from build123d import *

# Parameters (mm, degrees)
EXTRUDE_1_DEPTH = 2
EXTRUDE_2_DEPTH = 2
OTHER_START     = 1
OTHER_1_DEPTH   = 1


# Read off the part's stored shape, not the designer's step: Полость1
with BuildPart() as part:
    # Эскиз1 → Бобышка-Вытянуть1 (new body)
    with BuildSketch(Plane.XY):
        with BuildLine():
            Line((-4.017219652, 1.762254744), (-38.034439304, 16.684766311))
            ThreePointArc((-38.034439304, 16.684766311), (-46.743488079, 24.061279464), (-50, 35))
            Line((-50, 35), (-50, 150))
            Line((-50, 150), (50, 150))
            Line((50, 150), (50, 35))
            ThreePointArc((50, 35), (46.743488079, 24.061279464), (38.034439304, 16.684766311))
            Line((38.034439304, 16.684766311), (4.017219652, 1.762254744))
            ThreePointArc((4.017219652, 1.762254744), (0, 0.919871589), (-4.017219652, 1.762254744))
        make_face()
    extrude(amount=EXTRUDE_1_DEPTH)

    # Эскиз2 → Бобышка-Вытянуть2 (add)
    with BuildSketch(Plane.XY.offset(2)):
        with BuildLine():
            Line((50, 150), (-50, 150))
            Line((-50, 150), (-50, 35))
            ThreePointArc((-50, 35), (-46.743488079, 24.061279464), (-38.034439304, 16.684766311))
            Line((-38.034439304, 16.684766311), (-4.017219652, 1.762254744))
            ThreePointArc((-4.017219652, 1.762254744), (0, 0.919871589), (4.017219652, 1.762254744))
            Line((4.017219652, 1.762254744), (38.034439304, 16.684766311))
            ThreePointArc((38.034439304, 16.684766311), (46.743488079, 24.061279464), (50, 35))
            Line((50, 35), (50, 150))
        make_face()
        with BuildLine():
            Line((46, 146), (-46, 146))
            Line((-46, 146), (-46, 35))
            ThreePointArc((-46, 35), (-43.394790463, 26.249023571), (-36.427551443, 20.347813049))
            Line((-36.427551443, 20.347813049), (-2.410331791, 5.425301482))
            ThreePointArc((-2.410331791, 5.425301482), (0, 4.919871589), (2.410331791, 5.425301482))
            Line((2.410331791, 5.425301482), (36.427551443, 20.347813049))
            ThreePointArc((36.427551443, 20.347813049), (43.394790463, 26.249023571), (46, 35))
            Line((46, 35), (46, 146))
        make_face(mode=Mode.SUBTRACT)
    extrude(amount=EXTRUDE_2_DEPTH)

    # Полость1 outline → Полость1 (cut)
    with BuildSketch(Plane.XY.offset(OTHER_START)):
        with BuildLine():
            ThreePointArc((11.745635367, 75.156774095), (20.994280281, 69.854105541), (11.31836185, 65.378356547))
            ThreePointArc((11.31836185, 65.378356547), (5.115095453, 80.478737769), (3, 96.666029027))
            Line((3, 96.666029027), (4.5, 126.216029027))
            ThreePointArc((4.5, 126.216029027), (3.337458241, 132.579990058), (0, 138.121909927))
            ThreePointArc((0, 138.121909927), (-3.33745824, 132.579990058), (-4.5, 126.216029027))
            Line((-4.5, 126.216029027), (-3, 96.666029027))
            ThreePointArc((-3, 96.666029027), (-5.115095453, 80.478737769), (-11.31836185, 65.378356547))
            ThreePointArc((-11.31836185, 65.378356547), (-20.994280281, 69.854105541), (-11.745635367, 75.156774095))
            Line((-11.745635367, 75.156774095), (-13.469683479, 99.811810763))
            ThreePointArc((-13.469683479, 99.811810763), (-20.328911117, 119.444533663), (-36, 133.116029027))
            Line((-36, 133.116029027), (-36, 43.116029027))
            Line((-36, 43.116029027), (-16.549961479, 43.116029027))
            ThreePointArc((-16.549961479, 43.116029027), (-12.036010614, 31.549603352), (-3.567460781, 22.469866625))
            ThreePointArc((-3.567460781, 22.469866625), (-1.525407448, 20.507840011), (0, 18.121909927))
            ThreePointArc((0, 18.121909927), (1.525407448, 20.507840011), (3.567460781, 22.469866625))
            ThreePointArc((3.567460781, 22.469866625), (12.036010614, 31.549603352), (16.549961479, 43.116029027))
            Line((16.549961479, 43.116029027), (36, 43.116029027))
            Line((36, 43.116029027), (36, 133.116029027))
            ThreePointArc((36, 133.116029027), (20.328911117, 119.444533663), (13.469683479, 99.811810763))
            Line((13.469683479, 99.811810763), (11.745635367, 75.156774095))
        make_face()
        with BuildLine():
            ThreePointArc((-3, 29.83417227), (-7.667449376, 35.941229982), (-10.424893162, 43.116029027))
            Line((-10.424893162, 43.116029027), (-3, 43.116029027))
            Line((-3, 43.116029027), (-3, 29.83417227))
        make_face(mode=Mode.SUBTRACT)
        with BuildLine():
            ThreePointArc((-15.840643779, 58.145510324), (-16.78364457, 53.674469292), (-17.1, 49.116029027))
            Line((-17.1, 49.116029027), (-30, 49.116029027))
            Line((-30, 49.116029027), (-30, 67.116029027))
            Line((-30, 67.116029027), (-26.618950039, 67.116029027))
            ThreePointArc((-26.618950039, 67.116029027), (-22.676452369, 60.892576365), (-15.840643779, 58.145510324))
        make_face(mode=Mode.SUBTRACT)
        with BuildLine():
            ThreePointArc((-9.793333333, 57.413777048), (-4.715017619, 54.57423386), (-2.7, 49.116029027))
            Line((-2.7, 49.116029027), (-11.1, 49.116029027))
            ThreePointArc((-11.1, 49.116029027), (-10.771332925, 53.316029027), (-9.793333333, 57.413777048))
        make_face(mode=Mode.SUBTRACT)
        with BuildLine():
            Line((3, 29.83417227), (3, 43.116029027))
            Line((3, 43.116029027), (10.424893162, 43.116029027))
            ThreePointArc((10.424893162, 43.116029027), (7.667449376, 35.941229982), (3, 29.83417227))
        make_face(mode=Mode.SUBTRACT)
        with BuildLine():
            ThreePointArc((2.7, 49.116029027), (4.715017619, 54.57423386), (9.793333333, 57.413777048))
            ThreePointArc((9.793333333, 57.413777048), (10.771332925, 53.316029027), (11.1, 49.116029027))
            Line((11.1, 49.116029027), (2.7, 49.116029027))
        make_face(mode=Mode.SUBTRACT)
        with BuildLine():
            ThreePointArc((0, 79.005460407), (2.806605948, 70.695071551), (6.654810678, 62.812754617))
            ThreePointArc((6.654810678, 62.812754617), (3.005032266, 61.025332003), (0, 58.289359938))
            ThreePointArc((0, 58.289359938), (-3.005032266, 61.025332003), (-6.654810678, 62.812754617))
            ThreePointArc((-6.654810678, 62.812754617), (-2.806605948, 70.695071551), (0, 79.005460407))
        make_face(mode=Mode.SUBTRACT)
        with BuildLine():
            ThreePointArc((17.1, 49.116029027), (16.78364457, 53.674469292), (15.840643779, 58.145510324))
            ThreePointArc((15.840643779, 58.145510324), (22.676452369, 60.892576365), (26.618950039, 67.116029027))
            Line((26.618950039, 67.116029027), (30, 67.116029027))
            Line((30, 67.116029027), (30, 49.116029027))
            Line((30, 49.116029027), (17.1, 49.116029027))
        make_face(mode=Mode.SUBTRACT)
        with BuildLine():
            ThreePointArc((-18.216224905, 81.676993406), (-23.564060467, 78.521793021), (-26.618950039, 73.116029027))
            Line((-26.618950039, 73.116029027), (-30, 73.116029027))
            Line((-30, 73.116029027), (-30, 121.661547275))
            ThreePointArc((-30, 121.661547275), (-22.554855421, 111.225521288), (-19.413361995, 98.796851397))
            Line((-19.413361995, 98.796851397), (-18.216224905, 81.676993406))
        make_face(mode=Mode.SUBTRACT)
        with BuildLine():
            ThreePointArc((19.413361995, 98.796851397), (22.554855421, 111.225521288), (30, 121.661547275))
            Line((30, 121.661547275), (30, 73.116029027))
            Line((30, 73.116029027), (26.618950039, 73.116029027))
            ThreePointArc((26.618950039, 73.116029027), (23.564060467, 78.521793021), (18.216224905, 81.676993406))
            Line((18.216224905, 81.676993406), (19.413361995, 98.796851397))
        make_face(mode=Mode.SUBTRACT)
    extrude(amount=OTHER_1_DEPTH, mode=Mode.SUBTRACT)


solid = part.part
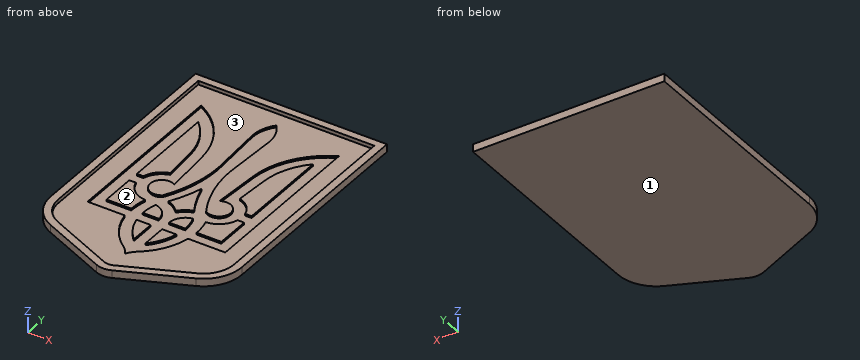
The model under review builds one solid part; all positions refer to its coordinate system, in mm. Face numbers are marked on the shaded views. Coordinates: 2 decimals unless noted, no trailing zeros. Order: outer loops, then holes, each group sorted by start corner. A loop starts at its lowest first (then second) coordinate and runs counter-clockwise, first axis right, second up. Notation, with made-up numbers: (87, 37.5) -> (117, 37.5) arc R32 ccw to (117, 71.5) -> close; hole circle Ø2 at (86, -40). An arc over 180 degrees is marked (long way). Answer in a Markdown table with one row per item.
(1) Consider section B-B (x = -33). Write out the cut boundary in (y, z).
Answers:
| item | result |
|---|---|
| outline | (14.48, 0) -> (150, 0) -> (150, 4) -> (146, 4) -> (146, 2) -> (131.47, 2) -> (131.47, 1) -> (43.12, 1) -> (43.12, 2) -> (18.84, 2) -> (18.84, 4) -> (14.48, 4) -> close |
(2) The part is to be moulded in two halves that separate along Y. For the marked faces 1, 2 and 3, say which applies: +Y half, -Y half, draft (parallel to the pull), parting line (faces both ways), or undercut.
Answers:
| item | result |
|---|---|
| face 1 | draft |
| face 2 | undercut |
| face 3 | undercut |
(3) Wall thickness on line 1 along X through (y, z) = (80.5, 2.35); line 2 along X through (y, z) = (59.5, 1.8); line 3 along X through (y, z) = (37, 1.85): over which ranges is each line inside the solid? List them lowest first.
Answers:
| item | result |
|---|---|
| line 1 | -50 to -46, 46 to 50 |
| line 2 | -50 to -36, -30 to -20.59, -1.12 to 1.12, 20.59 to 30, 36 to 50 |
| line 3 | -50 to -14.8, -8.23 to -3, 3 to 8.23, 14.8 to 50 |
(4) Consider section A-A (y = 41.5). Write out the cut boundary in (x, z), plus the area to 3 significant figures.
Answers:
| item | result |
|---|---|
| outline | (-50, 0) -> (50, 0) -> (50, 4) -> (46, 4) -> (46, 2) -> (16.21, 2) -> (16.21, 1) -> (10, 1) -> (10, 2) -> (3, 2) -> (3, 1) -> (-3, 1) -> (-3, 2) -> (-10, 2) -> (-10, 1) -> (-16.21, 1) -> (-16.21, 2) -> (-46, 2) -> (-46, 4) -> (-50, 4) -> close |
| area | 198 mm² |
(5) Insertion check: pin 1 (1.1 mm diameter, centred on x = 20.5, z = 1.5, fed in from -Y); pin 2 (11.5 mm diameter, centred on x = -22.5, y = 56.5, fed in from +Z); pin 3 (0.8 mm diameter, centred on x = -25, z = 1.5, fed in from -Y). Each pin has a flat end and moves straight along its axis. Give the tip position at first contact, or say it passes through.
Answers:
| item | result |
|---|---|
| pin 1 | y = 8.75 |
| pin 2 | z = 2 |
| pin 3 | y = 10.79 |
(6) Consider section C-C (y = 106). Write out the cut boundary in (x, z).
Answers:
| item | result |
|---|---|
| outline | (-50, 0) -> (50, 0) -> (50, 4) -> (46, 4) -> (46, 2) -> (36, 2) -> (36, 1) -> (30, 1) -> (30, 2) -> (20.63, 2) -> (20.63, 1) -> (14.43, 1) -> (14.43, 2) -> (3.47, 2) -> (3.47, 1) -> (-3.47, 1) -> (-3.47, 2) -> (-14.43, 2) -> (-14.43, 1) -> (-20.63, 1) -> (-20.63, 2) -> (-30, 2) -> (-30, 1) -> (-36, 1) -> (-36, 2) -> (-46, 2) -> (-46, 4) -> (-50, 4) -> close |
